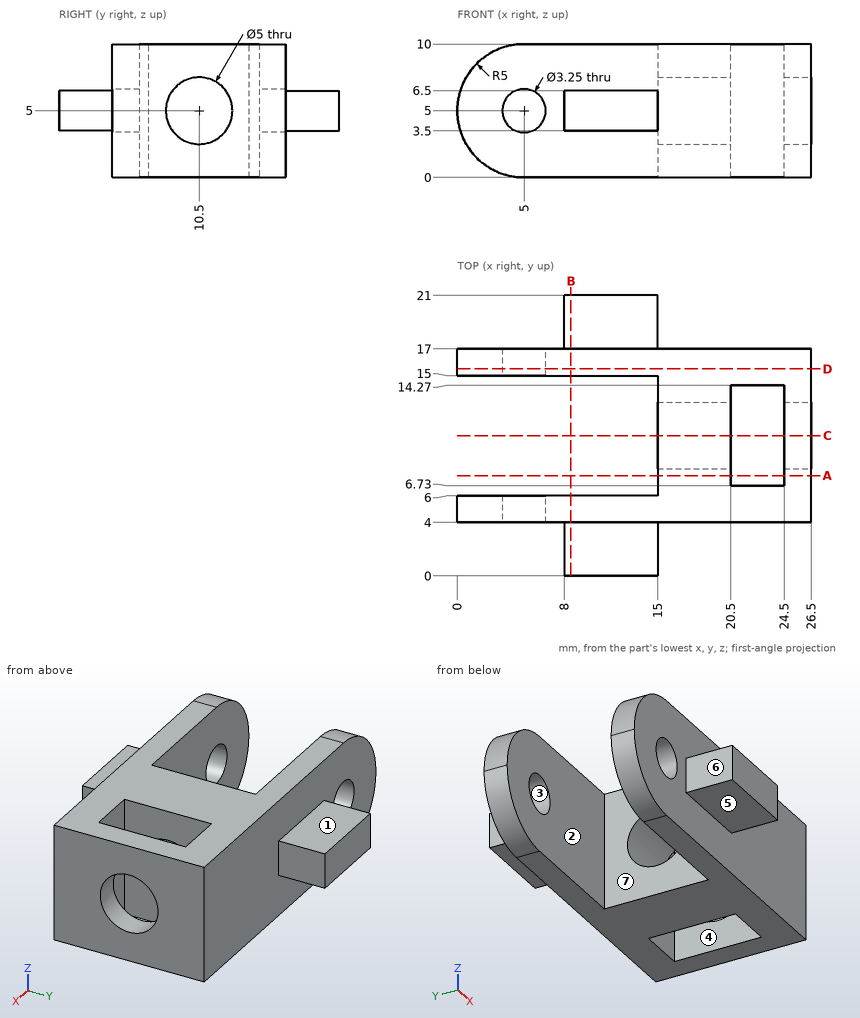
The figure shows three views and two pictorial views of one solid part (mm, origin at its lowest corner). Answer the questions. A direction names the side the tool comes from. Coordinates: 2 decimals unless noted, no trailing zeros. Loops run counter-clockwise (first coordinate to the right, second up) from the corner with the lowest first, then second, coordinate; pieces in that order, holes last. Notation, with made-up numbers: (33, 5.5) -> (50, 5.5) arc R18 ccw to (50, 12.5) -> close; hole circle Ø8 at (88.25, 55). An arc over 180 degrees is marked (long way). Return JSON: item names as keys, results as strings. Group by question number.
(1) Given pin 1 Ø1.5 at (y, z) = (2.5, 5) entering from -X; pin 2 Ø1.5 at (x, z) = (20, 2.5) entering from -Y; pin 3 Ø1.2 at (x, y) = (11, 19.5) entering from +Z, each flat-ended and moving along its own axis, determine where each tip first touches the part or whether it passes through.
(2) A cutting plane is placed at A-A on y = 7.5. Write down the section's boundary in (x, z).
(3) A cutting plane is placed at D-D on y = 15.5. Write down the section's boundary in (x, z) (3 decimals), and give its area (3 significant figures).
(4) A cutting plane is placed at C-C on y = 10.5. Write down the section's boundary in (x, z), and give its area (3 significant figures).
(5) Which of the six approach directions +Z, -Z, +X, -X, +Y, -Y give full straight-line access (tool end or side, diameter ignored) to the marked faces 4, 5, 6 and 7?
(6) Determine the mould class of the marked faces 1, 2 and 3 for opening direction Z: released by +Z, released by -Z, zero draft, split by the parting line, or undercut.
(7) A cutting plane is placed at B-B on x = 8.5. Write down the section's boundary in (y, z).
(8) Find the intervals of material crossed by probe 1 along Y at (x, z) = (8.5, 7.5); probe 2 along X at (y, z) = (11.25, 8); probe 3 along Y at (x, z) = (14.75, 4.5), in increasing order. Write a range as from..to.
The answers:
{
 "1": {"pin 1": "stops at x = 8", "pin 2": "stops at y = 4", "pin 3": "stops at z = 6.5"},
 "2": {"outline": "(15, 0) -> (20.5, 0) -> (20.5, 10) -> (15, 10) -> close; (24.5, 0) -> (26.5, 0) -> (26.5, 10) -> (24.5, 10) -> close"},
 "3": {"outline": "(5, 0) -> (26.5, 0) -> (26.5, 10) -> (5, 10) arc R5 ccw to start; hole circle Ø3.25 at (5, 5)", "area": "246 mm^2"},
 "4": {"outline": "(15, 0) -> (20.5, 0) -> (20.5, 2.5) -> (15, 2.5) -> close; (15, 7.5) -> (20.5, 7.5) -> (20.5, 10) -> (15, 10) -> close; (24.5, 0) -> (26.5, 0) -> (26.5, 2.5) -> (24.5, 2.5) -> close; (24.5, 7.5) -> (26.5, 7.5) -> (26.5, 10) -> (24.5, 10) -> close", "area": "37.5 mm^2"},
 "5": {"face 4": "+Z, -Z", "face 5": "-Z, +X, -X, -Y", "face 6": "+Z, -Z, -X, -Y", "face 7": "+Z, -Z, -X"},
 "6": {"face 1": "released by +Z", "face 2": "zero draft", "face 3": "undercut"},
 "7": {"outline": "(0, 3.5) -> (4, 3.5) -> (4, 0) -> (6, 0) -> (6, 10) -> (4, 10) -> (4, 6.5) -> (0, 6.5) -> close; (15, 0) -> (17, 0) -> (17, 3.5) -> (21, 3.5) -> (21, 6.5) -> (17, 6.5) -> (17, 10) -> (15, 10) -> close"},
 "8": {"probe 1": "y = 4..6, 15..17", "probe 2": "x = 15..20.5, 24.5..26.5", "probe 3": "y = 0..6, 15..21"}
}
